Verification items for the finished model (mm, model axes). A direction names the side the tool comes from. Coordinates: 2 decimals unless noted, no trailing zeros. Loops run counter-clockwise (first coordinate to the right, second up) from the corner with the lowest first, then second, coordinate; pieces in that order, holes last. Notation, with made-up numbers: (-4, 13.25) - (40, 13.25) arc R22 cw to (40, 25.25) - close; hole circle Ø1 at (30.5, -4.5). An arc over 180 degrees is marked (long way). One line per item, written item: value. Start each with the question number.
(1) Section check D-D (z = -9.5). Record the boundary of the cut face in (x, y).
(2) Section check A-A (z = -13.75). Record the boundary of the cut face in (x, y), plus the area to 3 significant figures.
(3) Set-up check for faces 1 (the face through (-8.118, -19.629, -14.477)), 2 (the face through (-9, -38.717, -10)): record each of +Z, -Z, +X, -X, +Y, -Y from which the full face is reachable in a straight line by a thin tool's end or side.
(4) Section check B-B (x = -10.25). Record the boundary of the cut face in (y, z).
(5) Section check C-C (y = -18.5). Record the boundary of the cut face in (x, z), plus the area to 3 significant figures.
(6) Thickness scan on probe 1 along Y at (x, z) = (-11.25, -2.5); probe 2 along Z at (x, y) = (-16, 23.5); probe 3 along Y at (x, z) = (-12.75, -14.5). Record the ranges inside material, lowest first. Write a range as [from, to].
(7) Gauge pin test, flat ends, axial feed: P1, Ø2, axis at x = -13, y = -12.5, coming from the -Z side; P2, Ø10, axis at x = -7, y = -24.5, coming from the -Z side; P3, Ø6, axis at y = -17.5, z = -14.5, coming from the +X side. Record the tip position at first contact, or that the pin passes through.
```python
from build123d import *

# Parameters (mm, degrees)
SKETCH1_W           = 17.751360412
SKETCH1_H           = 20.289442188
BOSS_EXTRUDE1_DEPTH = 40
SKETCH2_R           = 3.980814887
CUT_EXTRUDE1_DEPTH  = 40


with BuildPart() as part:
    # Sketch1 → Boss-Extrude1 (new body)
    with BuildSketch(Plane(origin=(0, 0, 0), x_dir=(1, 0, 0), z_dir=(0, 1, 0))):
        with Locations((-8.875680206, 10.144721094)):
            Rectangle(SKETCH1_W, SKETCH1_H)
    extrude(amount=BOSS_EXTRUDE1_DEPTH)

    # Sweep1: sweep along a curve in space
    with BuildLine() as sweep1_path:
        Line((-8.636006498, 0, -10.530435866), (-8.636006498, -38.716526094, -10.530435866))
    # Sketch2 → Sweep1 (sweep)
    with BuildSketch(Plane(origin=(0, 0, 0), x_dir=(-1, 0, 0), z_dir=(0, -1, 0))):
        with Locations((8.636006498, 10.530435866)):
            Circle(SKETCH2_R)
    sweep(path=sweep1_path.line)

    # Sketch3 → Cut-Extrude1 (cut)
    with BuildSketch(Plane(origin=(0, 0, 0), x_dir=(0, 0, -1), z_dir=(1, 0, 0))):
        Polygon((27.331751958, 3.526611328), (13.036737594, 14.826732859), (11.549169686, 44.474117194), (29.802797672, 42.721399119), align=None)
    extrude(amount=-CUT_EXTRUDE1_DEPTH, mode=Mode.SUBTRACT)


solid = part.part
```
Responses:
1. outline: (-17.75, 0) - (-12.48, 0) - (-12.48, -38.72) - (-4.79, -38.72) - (-4.79, 0) - (0, 0) - (0, 40) - (-17.75, 40) - close
2. outline: (-17.75, 0) - (-10.98, 0) - (-10.98, -38.72) - (-6.29, -38.72) - (-6.29, 0) - (0, 0) - (0, 14.26) - (-17.75, 14.26) - close
2. area: 434 mm²
3. face 1: -Y
3. face 2: +Z, -Z, +X, -X, -Y
4. outline: (-38.72, -14.17) - (0, -14.17) - (0, -20.29) - (9.09, -20.29) - (14.83, -13.04) - (40, -11.77) - (40, 0) - (0, 0) - (0, -6.89) - (-38.72, -6.89) - close
5. outline: circle Ø7.96 at (-8.64, -10.53)
5. area: 49.8 mm²
6. probe 1: y = [0, 40]
6. probe 2: z = [-12.6, 0]
6. probe 3: y = [0, 13.67]
7. P1: stops at z = -12.66
7. P2: stops at z = -14.51
7. P3: stops at x = -4.78
